Geometry: final body of the model. Coordinates: model frame, mm. A direction names the side the tool comes from. Round coordinates to 2 decimals unless told otherwise and drop trailing zeros. Loops run counter-clockwise (first coordinate to the right, second up) from the corner with the lowest first, then second, coordinate; pieces in that order, holes last. Notation, with made-up numbers: (9.5, 1.5) - (27.5, 1.5) arc R16 cw to (27.5, 28.5) - close; hole circle Ø8 at (17.5, 11.5). An arc over 180 degrees is marked (long way). Answer as CSV lines item,"result".
from build123d import *

# Parameters (mm, degrees)
PAD_DEPTH       = 6.5
SKETCH001_W     = 27
SKETCH001_H     = 6
SKETCH001_W_2   = 6
SKETCH001_H_2   = 27
PAD001_DEPTH    = 1
SKETCH002_R     = 1.6
POCKET_DEPTH    = 7.501
SKETCH003_R     = 3
POCKET001_DEPTH = 1


with BuildPart() as part:
    # Sketch → Pad (new body)
    with BuildSketch(Plane.XY):
        with BuildLine():
            Line((-9.5, 40.5), (9.5, 40.5))
            Line((9.5, 40.5), (9.5, -9.5))
            Line((9.5, -9.5), (-40.5, -9.5))
            Line((-40.5, -9.5), (-40.5, 9.5))
            Line((-40.5, 9.5), (-18.5, 9.5))
            ThreePointArc((-18.5, 9.5), (-12.136039, 12.136039), (-9.5, 18.5))
            Line((-9.5, 18.5), (-9.5, 40.5))
        make_face()
    extrude(amount=PAD_DEPTH)

    # Sketch001 → Pad001 (new body)
    with BuildSketch(Plane(origin=(0, 0, 0), x_dir=(1, 0, 0), z_dir=(0, 0, -1))):
        with Locations((-25, 0)):
            Rectangle(SKETCH001_W, SKETCH001_H)
        with Locations((0, -25)):
            Rectangle(SKETCH001_W_2, SKETCH001_H_2)
    extrude(amount=PAD001_DEPTH)

    # Sketch002 → Pocket (cut, through all)
    with BuildSketch(Plane.XY.offset(6.5)):
        with Locations((-33.5, 0)):
            Circle(SKETCH002_R)
        with Locations((-15.5, 0)):
            Circle(SKETCH002_R)
        with Locations((0, 15.5)):
            Circle(SKETCH002_R)
        with Locations((0, 33.5)):
            Circle(SKETCH002_R)
    extrude(amount=-POCKET_DEPTH, mode=Mode.SUBTRACT)

    # Sketch003 → Pocket001 (cut)
    with BuildSketch(Plane.XY.offset(6.5)):
        with Locations((3, 11.5)):
            Circle(SKETCH003_R)
        with Locations((-12.5, 0)):
            Circle(SKETCH003_R)
        with Locations((-36.376617, 5.782363)):
            Circle(SKETCH003_R)
        with Locations((-27, 2.406107)):
            Circle(SKETCH003_R)
    extrude(amount=-POCKET001_DEPTH, mode=Mode.SUBTRACT)


solid = part.part
(1) Section D-D (x = -1). Output: boundary loops of the cut face in (y, z).
Findings below:
outline,"(-9.5, 0) - (11.5, 0) - (11.5, -1) - (14.25, -1) - (14.25, 6.5) - (-9.5, 6.5) - close; (16.75, -1) - (32.25, -1) - (32.25, 6.5) - (16.75, 6.5) - close; (34.75, -1) - (38.5, -1) - (38.5, 0) - (40.5, 0) - (40.5, 6.5) - (34.75, 6.5) - close"
(2) Access query for faces 5 (the face through (-12, 0, 5.5)), 6 (the face through (-10, 10, 6.5)), 7 (the face through (-30, 9.5, 3)). Directions: +Z, -Z, +X, -X, +Y, -Y. A direction counts if a zero-diameter tool reaches every point of the face in a straight line with its end or side. Return the directions, or none.
Findings below:
face 5,"+Z"
face 6,"+Z, +X, -X, +Y, -Y"
face 7,"+Z, -Z, -X, +Y"
(3) Pin query (flat end, axial travel): P1, Ø1.5, axis at x = -18.5, z = 0.5, coming from the +Y side; P2, Ø0.8, axis at x = -24.5, z = -0.5, coming from the +Y side; P3, Ø1.9, axis at x = -15.5, y = 0, coming from the -Z side; P4, Ø0.5, axis at x = 0.5, z = -0.5, coming from the +Y side. Return the tip coordinate at first contact, or that it passes through.
Findings below:
P1,"y = 9.53"
P2,"y = 3"
P3,"through"
P4,"y = 38.5"
(4) Draft query along X for faces 1 (the face through (9.5, 16, 3)), 2 (the face through (0, 25, -1)), 3 (the face through (-33.515, 6.683, 6.007)), 4 (the face through (-12.206, 12.066, 3.204)). Return one class per face: pulls with the +X half, pulls with the -X half, needs draft (parallel to the pull), parting line crosses it, or undercut.
Findings below:
face 1,"pulls with the +X half"
face 2,"needs draft"
face 3,"undercut"
face 4,"pulls with the -X half"
(5) Section C-C (y = 0). Output: boundary loops of the cut face in (x, z), and give its area (3 significant figures).
Findings below:
outline,"(-40.5, 0) - (-38.5, 0) - (-38.5, -1) - (-35.1, -1) - (-35.1, 6.5) - (-40.5, 6.5) - close; (-31.9, -1) - (-17.1, -1) - (-17.1, 6.5) - (-25.21, 6.5) - (-25.21, 5.5) - (-28.79, 5.5) - (-28.79, 6.5) - (-31.9, 6.5) - close; (-13.9, -1) - (-11.5, -1) - (-11.5, 0) - (9.5, 0) - (9.5, 6.5) - (-9.5, 6.5) - (-9.5, 5.5) - (-13.9, 5.5) - close"
area,"296 mm2"
(6) Material intervals for line 1 along Y through (x, z) = (0, 2.5); line 2 along Y through (x, z) = (3, 5.75); line 3 along Y through (x, z) = (-27, 5.7), sorted ascending.
Findings below:
line 1,"-9.5 to 13.9, 17.1 to 31.9, 35.1 to 40.5"
line 2,"-9.5 to 8.5, 14.5 to 40.5"
line 3,"-9.5 to -0.59, 5.41 to 9.5"
(7) Section A-A (z = 2.25). Output: boundary loops of the cut face in (x, y), and give its area (3 significant figures).
Findings below:
outline,"(-40.5, -9.5) - (9.5, -9.5) - (9.5, 40.5) - (-9.5, 40.5) - (-9.5, 18.5) arc R9 cw to (-18.5, 9.5) - (-40.5, 9.5) - close; hole circle Ø3.2 at (-33.5, 0); hole circle Ø3.2 at (-15.5, 0); hole circle Ø3.2 at (0, 15.5); hole circle Ø3.2 at (0, 33.5)"
area,"1,520 mm2"
(8) Section B-B (x = -16.5). Output: boundary loops of the cut face in (y, z), and give its area (3 significant figures).
Findings below:
outline,"(-9.5, 0) - (-3, 0) - (-3, -1) - (-1.25, -1) - (-1.25, 6.5) - (-9.5, 6.5) - close; (1.25, -1) - (3, -1) - (3, 0) - (9.73, 0) - (9.73, 6.5) - (1.25, 6.5) - close"
area,"112 mm2"
